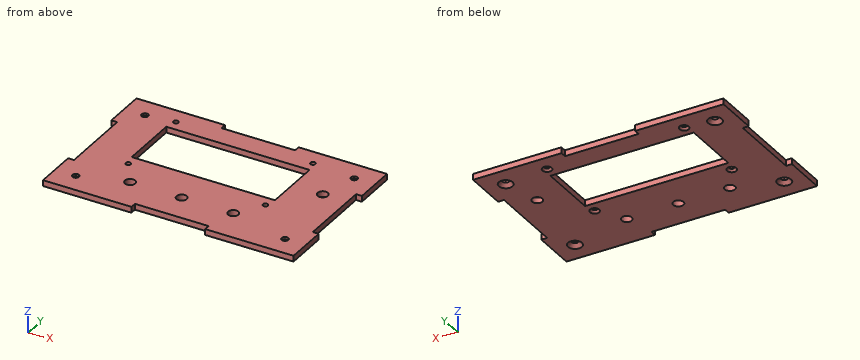
```python
from build123d import *

# Parameters (mm, degrees)
SKETCH1_W                                    = 170
SKETCH1_H                                    = 108
PLATE_DEPTH                                  = 4
SKETCH2_W                                    = 97.2
SKETCH2_H                                    = 40
SCREEN_SLOT_DEPTH                            = 101.781942827
SCREEN_SCREW_HOLES_D                         = 3.4
SCREEN_SCREW_HOLES_CSINK_D                   = 6.3
SCREEN_SCREW_HOLES_CSINK_ANGLE               = 90
KNOB_HOLES_D                                 = 7
CUT_EXTRUDE2_REACH                           = 102.782
SKETCH8_W                                    = 50
SKETCH8_H                                    = 4
SKETCH8_W_2                                  = 4
SKETCH8_H_2                                  = 50
CSK_FOR_M4_COUNTERSUNK_FLAT_HEAD_SCR_2_COUNT = 2
CSK_FOR_M4_COUNTERSUNK_FLAT_HEAD_SCR_2_PITCH = 142
CSK_FOR_M4_COUNTERSUNK_FLAT_HEAD_SCR_3_COUNT = 2
CSK_FOR_M4_COUNTERSUNK_FLAT_HEAD_SCR_3_PITCH = 162.984661855
CSK_FOR_M4_COUNTERSUNK_FLAT_HEAD_SCR_4_COUNT = 2
CSK_FOR_M4_COUNTERSUNK_FLAT_HEAD_SCR_4_PITCH = 80


with BuildPart() as part:
    # Sketch1 → Plate (new body)
    with BuildSketch(Plane.XY):
        Rectangle(SKETCH1_W, SKETCH1_H)
    extrude(amount=PLATE_DEPTH)

    # Sketch2 → Screen slot (cut, through all)
    with BuildSketch(Plane(origin=(0, 0, 0), x_dir=(-1, 0, 0), z_dir=(0, 0, -1))):
        with Locations((5, 15)):
            Rectangle(SKETCH2_W, SKETCH2_H)
    extrude(amount=-SCREEN_SLOT_DEPTH, mode=Mode.SUBTRACT)

    # Screen screw holes (through all)
    with Locations(Plane(origin=(41.5, 42.5, 0), x_dir=(-1, 0, 0), z_dir=(0, 0, -1))):
        with Locations((0, 0), (93, 0), (93, -55), (0, -55)):
            CounterSinkHole(SCREEN_SCREW_HOLES_D / 2, SCREEN_SCREW_HOLES_CSINK_D / 2, counter_sink_angle=SCREEN_SCREW_HOLES_CSINK_ANGLE)

    # Knob holes (through all)
    with Locations(Plane(origin=(30, -30, 0), x_dir=(-1, 0, 0), z_dir=(0, 0, -1))):
        with Locations((0, 0), (35, 0), (70, 0), (-34.3, 45)):
            Hole(KNOB_HOLES_D / 2)

    # Sketch8 → Cut-Extrude2 (cut, up to next)
    with BuildSketch(Plane(origin=(0, 0, 0), x_dir=(-1, 0, 0), z_dir=(0, 0, -1)), mode=Mode.PRIVATE) as cut_extrude2_sk1:
        with Locations((0, 52)):
            Rectangle(SKETCH8_W, SKETCH8_H)
    cut_extrude2_tool1 = extrude(cut_extrude2_sk1.sketch, amount=-CUT_EXTRUDE2_REACH, mode=Mode.PRIVATE) & part.part
    # Sketch8 → Cut-Extrude2 (cut, up to next)
    with BuildSketch(Plane(origin=(0, 0, 0), x_dir=(-1, 0, 0), z_dir=(0, 0, -1)), mode=Mode.PRIVATE) as cut_extrude2_sk2:
        with Locations((83, 0)):
            Rectangle(SKETCH8_W_2, SKETCH8_H_2)
    cut_extrude2_tool2 = extrude(cut_extrude2_sk2.sketch, amount=-CUT_EXTRUDE2_REACH, mode=Mode.PRIVATE) & part.part
    # Sketch8 → Cut-Extrude2 (cut, up to next)
    with BuildSketch(Plane(origin=(0, 0, 0), x_dir=(-1, 0, 0), z_dir=(0, 0, -1)), mode=Mode.PRIVATE) as cut_extrude2_sk3:
        with Locations((0, -52)):
            Rectangle(SKETCH8_W, SKETCH8_H)
    cut_extrude2_tool3 = extrude(cut_extrude2_sk3.sketch, amount=-CUT_EXTRUDE2_REACH, mode=Mode.PRIVATE) & part.part
    # Sketch8 → Cut-Extrude2 (cut, up to next)
    with BuildSketch(Plane(origin=(0, 0, 0), x_dir=(-1, 0, 0), z_dir=(0, 0, -1)), mode=Mode.PRIVATE) as cut_extrude2_sk4:
        with Locations((-83, 0)):
            Rectangle(SKETCH8_W_2, SKETCH8_H_2)
    cut_extrude2_tool4 = extrude(cut_extrude2_sk4.sketch, amount=-CUT_EXTRUDE2_REACH, mode=Mode.PRIVATE) & part.part
    add(cut_extrude2_tool1.solids().sort_by_distance((0, 52, 0))[0], mode=Mode.SUBTRACT)
    add(cut_extrude2_tool2.solids().sort_by_distance((-83, 0, 0))[0], mode=Mode.SUBTRACT)
    add(cut_extrude2_tool3.solids().sort_by_distance((0, -52, 0))[0], mode=Mode.SUBTRACT)
    add(cut_extrude2_tool4.solids().sort_by_distance((83, 0, 0))[0], mode=Mode.SUBTRACT)

    # Sketch10 → CSK for M4 Countersunk Flat Head Screw1 (revolve, cut)
    with BuildSketch(Plane(origin=(71, 40, 0), x_dir=(0, 1, 0), z_dir=(1, 0, 0))):
        Polygon((0, 0), (0, 4), (2.25, 4), (2.25, 2.45), (4.7, 0), align=None)
    csk_for_m4_countersunk_flat_head_screw1 = revolve(axis=Axis((71, 40, -6.35), (0, 0, 1)), mode=Mode.SUBTRACT)

    # CSK for M4 Countersunk Flat Head Scr 2: CSK for M4 Countersunk Flat Head Screw1 ×2
    with Locations(*[(-i * CSK_FOR_M4_COUNTERSUNK_FLAT_HEAD_SCR_2_PITCH, 0, 0) for i in range(1, CSK_FOR_M4_COUNTERSUNK_FLAT_HEAD_SCR_2_COUNT)]):
        add(csk_for_m4_countersunk_flat_head_screw1, mode=Mode.SUBTRACT)

    # CSK for M4 Countersunk Flat Head Scr 3: CSK for M4 Countersunk Flat Head Screw1 ×2
    with Locations(*[Vector(-0.8712476277448776, -0.49084373394077596, 0) * (i * CSK_FOR_M4_COUNTERSUNK_FLAT_HEAD_SCR_3_PITCH) for i in range(1, CSK_FOR_M4_COUNTERSUNK_FLAT_HEAD_SCR_3_COUNT)]):
        add(csk_for_m4_countersunk_flat_head_screw1, mode=Mode.SUBTRACT)

    # CSK for M4 Countersunk Flat Head Scr 4: CSK for M4 Countersunk Flat Head Screw1 ×2
    with Locations(*[(0, -i * CSK_FOR_M4_COUNTERSUNK_FLAT_HEAD_SCR_4_PITCH, 0) for i in range(1, CSK_FOR_M4_COUNTERSUNK_FLAT_HEAD_SCR_4_COUNT)]):
        add(csk_for_m4_countersunk_flat_head_screw1, mode=Mode.SUBTRACT)


solid = part.part
```
Build history of the part. All positions in model axes, mm. Round coordinates to 2 decimals unless told otherwise and drop trailing zeros. Loops run counter-clockwise (first coordinate to the right, second up) from the corner with the lowest first, then second, coordinate; pieces in that order, holes last. Notation, with made-up numbers: M 7.25,55 L 20.25,55 A11 ccw 20.25,68 Z; hole C -21.75,-1.75 d4. An arc over 180 degrees is marked long. Answer as CSV lines item,"result".
1. Cut at D-D on x = 41.5. Write the cut outline in (y, z), then the cut area to 3 significant figures.
Resolved:
outline,"M -54,0 L -15.65,0 L -14.2,1.45 L -14.2,4 L -54,4 Z; M -10.8,1.45 L -9.35,0 L -5,0 L -5,4 L -10.8,4 Z; M 35,0 L 39.35,0 L 40.8,1.45 L 40.8,4 L 35,4 Z; M 44.2,1.45 L 45.65,0 L 54,0 L 54,4 L 44.2,4 Z"
area,"241 mm²"
2. Cut at C-C on x = 11.5. Write the cut outline in (y, z), then the cut area to 3 significant figures.
Resolved:
outline,"M -50,0 L -5,0 L -5,4 L -50,4 Z; M 35,0 L 50,0 L 50,4 L 35,4 Z"
area,"240 mm²"
3. Cut at A-A on x = -71. Write the cut outline in (y, z).
Resolved:
outline,"M -54,0 L -44.7,0 L -42.25,2.45 L -42.25,4 L -54,4 Z; M -37.75,2.45 L -35.3,0 L 35.3,0 L 37.75,2.45 L 37.75,4 L -37.75,4 Z; M 42.25,2.45 L 44.7,0 L 54,0 L 54,4 L 42.25,4 Z"
4. Cut at B-B on y = -40. Write the cut outline in (x, z), then the cut area to 3 significant figures.
Resolved:
outline,"M -85,0 L -75.7,0 L -73.25,2.45 L -73.25,4 L -85,4 Z; M -68.75,2.45 L -66.3,0 L 66.3,0 L 68.75,2.45 L 68.75,4 L -68.75,4 Z; M 73.25,2.45 L 75.7,0 L 85,0 L 85,4 L 73.25,4 Z"
area,"632 mm²"
5. Flat gauge pins, fed straight in: P1, Ø3, axis at x = 55.5, y = 17.5, coming from the -Z side; P2, Ø2, axis at y = 13, z = 1, coming from the -X side; P3, Ø2, axis at x = -18, z = 1.5, coming from the -Y side. Where does each tip first touch, or does it go through?
Resolved:
P1,"stops at z = 0"
P2,"stops at x = -81"
P3,"stops at y = -50"
6. Wall check: probe 1 along X at (y, z) = (-12.5, 2.7); probe 2 along Y at (x, z) = (30, 1.7); probe 3 along X at (y, z) = (-40, 2.9). Give the ranges that are in metal, low to high. Write a range as [from, to].
Resolved:
probe 1,"x = [-81, -53.2], [-49.8, 39.8], [43.2, 81]"
probe 2,"y = [-54, -33.5], [-26.5, -5], [35, 54]"
probe 3,"x = [-85, -73.25], [-68.75, 68.75], [73.25, 85]"
